Geometry check sheet. Reference: the model listing, model coordinates, mm. A direction names the side the tool comes from. Give positions to 0.01 mm unless a question says otherwise; leave off trailing zeros. Order: outer loops, then holes, each group sorted by start corner. A loop starts at its lowest first (then second) coordinate and runs counter-clockwise, first axis right, second up.
```python
from build123d import *

# Parameters (mm, degrees)
F_2020_SKETCH_R     = 3
BOSS_EXTRUDE1_DEPTH = 100


with BuildPart() as part:
    # 2020 sketch → Boss-Extrude1 (new body)
    with BuildSketch(Plane(origin=(0, 0, 0), x_dir=(1, 0, 0), z_dir=(0, 1, 0))):
        Polygon((-4, 10), (-4, 8), (-7, 8), (-3, 4), (3, 4), (7, 8), (4, 8), (4, 10), (10, 10), (10, 4), (8, 4), (8, 7), (4, 3), (4, -3), (8, -7), (8, -4), (10, -4), (10, -10), (4, -10), (4, -8), (7, -8), (3, -4), (-3, -4), (-7, -8), (-4, -8), (-4, -10), (-10, -10), (-10, -4), (-8, -4), (-8, -7), (-4, -3), (-4, 3), (-8, 7), (-8, 4), (-10, 4), (-10, 10), align=None)
        Circle(F_2020_SKETCH_R, mode=Mode.SUBTRACT)
    boss_extrude1 = extrude(amount=BOSS_EXTRUDE1_DEPTH)

    # Mirror1: Boss-Extrude1 across plane
    add(boss_extrude1.mirror(Plane(origin=(10, 100, 4), x_dir=(0, 0, 1), z_dir=(1, 0, 0))))


solid = part.part
```
Q1. Cross-section at A-A, the plane z = 0. Record the boundary of the cut face in (x, y), and give its area (3 significant figures).
Q2. Cross-section at B-B, the plane x = 11. Record the boundary of the cut face in (y, z).
Q3. Release check for a two-part mould opening along Z. For faces 4 (the face through (-7, 49, -10)), 5 (the face through (26, 49, 8)), 6 (the face through (24, 49, 9)) record: pulls with the +Z half, pulls with the -Z half, needs draft (parallel to the pull), parting line crosses it, or undercut.
Q4. Gauge pin test, flat ends, axial feed: P1, Ø6.5, axis at y = 61, z = -0.5, coming from the -X side; P2, Ø3, axis at x = 21, y = 23.5, coming from the +Z side; P3, Ø1.5, axis at y = 52, z = 1.5, coming from the -X side. Record the tip position at first contact, or that the pin passes through.
Q5. Thickness scan on L1, parallel to X at y = 29, z = 0; L2, parallel to X at y = 87, z = 8.5; L3, parallel to X at y = 55, z = 1.5. Record the ranges inside material, lowest first.
Q6. Access from +Z, -Z, +X, -X, +Y, -Y to the whole of each face (thin tool, end or side, straight path). Record for faces 1 (the face through (24, 49, -9)), 2 (the face through (4, 49, 9)), 3 (the face through (10, 49, -4)).
Q7. Cross-section at D-D, the plane y = 34.5. Give the number of separate pieces and of enclosed holes in the cut face, and give its area (3 significant figures).
Q8. Cross-section at C-C, the plane x = 0. Record the boundary of the cut face in (y, z), and give its area (3 significant figures).
Answers follow:
1. outline: (-4, 0) - (-3, 0) - (-3, 100) - (-4, 100) - close; (3, 0) - (4, 0) - (4, 100) - (3, 100) - close; (16, 0) - (17, 0) - (17, 100) - (16, 100) - close; (23, 0) - (24, 0) - (24, 100) - (23, 100) - close
1. area: 400 mm2
2. outline: (0, -10) - (100, -10) - (100, -4) - (0, -4) - close; (0, 4) - (100, 4) - (100, 10) - (0, 10) - close
3. face 4: pulls with the -Z half
3. face 5: undercut
3. face 6: needs draft
4. P1: stops at x = -4.75
4. P2: stops at z = 4
4. P3: stops at x = -4
5. L1: x = -4 to -3, 3 to 4, 16 to 17, 23 to 24
5. L2: x = -10 to -4, 4 to 16, 24 to 30
5. L3: x = -4 to -2.6, 2.6 to 4, 16 to 17.4, 22.6 to 24
6. face 1: -Z, +Y, -Y
6. face 2: +Z, +Y, -Y
6. face 3: +Y, -Y
7. separate pieces: 1
7. enclosed holes: 3
7. area: 295 mm2
8. outline: (0, -4) - (100, -4) - (100, -3) - (0, -3) - close; (0, 3) - (100, 3) - (100, 4) - (0, 4) - close
8. area: 200 mm2
